Here's how the part is built. I have some questions about the finished solid (model axes, mm). A direction names the side the tool comes from. Coordinates: 2 decimals unless noted, no trailing zeros. Write each loop counter-clockwise with the first axis right and the second up, starting at its lowest first coordinate (ties: lowest second). Pieces come first, ordered by that corner, then holes. Notation, with made-up numbers: (54.5, -30) -> (68.5, -30) arc R13 ccw to (68.5, -20) -> close; hole circle Ø1 at (-1.5, -28). An arc over 180 degrees is marked (long way). Put each result on its own line as item: value. Start each with the question number.
Item 1: If we mould it in two halves opening along Y, with no side actions, what happens to faces 1 (the face through (70.768, -13.596, 0.044)), 2 (the face through (0, -9.8, 27)), 3 (the face through (1, 6, -3.175))? For each: released by +Y, released by -Y, zero draft, split by the parting line, or undercut.
Item 2: For pin 1 (9 mm diameter, centred on x = 58.5, y = -11.5, fed in from +Z) (3 decimals); pin 2 (2 mm diameter, centred on x = 60, z = 3, fed in from +Y); pin 3 (2.5 mm diameter, centred on x = 49, y = 33, fed in from +Z) (3 decimals); pin 4 (12 mm diameter, centred on x = 60.325, y = 18.775, fed in from +Z), each with a flat end and sliding along its axis, tell me the tip position at first contact or that it passes through.
Item 3: On a 3-axis mill with a long thin cutter (end or side, diameter ignored), from which of +Z, -Z, +X, -X, +Y, -Y can I reach the whole of each face in a straight line? I mean faces 4 (the face through (59, -10, 0.875)), 5 (the face through (75.59, 10.04, -1.89)), 6 (the face through (-6.133, -14.629, 25.39)). Say none if no direction works.
Item 4: I want a section at A-A, the plane z = 7. List the corners of the cut face in (x, y) for me (3 decimals).
Item 5: I want a section at B-B, the plane x = 0. List the corners of the cut face in (y, z) for me (1 decimal), then the cut area to 3 significant figures.
Item 6: I need wall thicknesses on line 1 (X direction, y = -9, z = -1); line 2 (X direction, y = -17, z = 25); line 3 (Z direction, x = 21, y = -13) (3 decimals). Which ranges of each line are inside material? Lowest first, please. Write a range as [from, to].
from build123d import *

# Parameters (mm, degrees)
BOSS_EXTRUDE1_DEPTH                              = 3.175
SKETCH2_W                                        = 31.75
SKETCH2_H                                        = 9.525
BOSS_EXTRUDE2_DEPTH                              = 47.419999902
SKETCH3_R                                        = 1.5
CUT_EXTRUDE1_DEPTH                               = 12.7
SKETCH6_R                                        = 1.5
CUT_EXTRUDE2_DEPTH                               = 12.7
SKETCH7_R                                        = 1.5
CUT_EXTRUDE3_DEPTH                               = 12.7
FILLET1_R                                        = 9.525
SKETCH12_R                                       = 7.5
CUT_EXTRUDE4_DEPTH                               = 101.032629802
CUT_EXTRUDE5_START                               = -2.54
CUT_EXTRUDE5_DEPTH                               = 2.54
FILLET3_R                                        = 1.5875
FILLET3_OF_MIRROR2_R                             = 1.5875
CBORE_FOR_M3_HEX_HEAD_MACHINE_SCREW1_D           = 3.4
CBORE_FOR_M3_HEX_HEAD_MACHINE_SCREW1_CBORE_D     = 8.4
CBORE_FOR_M3_HEX_HEAD_MACHINE_SCREW1_CBORE_DEPTH = 2.3
SKETCH19_R                                       = 4.7625
CUT_EXTRUDE6_DEPTH                               = 101.032629802


with BuildPart() as part:
    # Sketch1 → Boss-Extrude1 (new, symmetric)
    with BuildSketch(Plane.XY):
        with BuildLine():
            Line((-57.15, 44.175), (57.15, 44.175))
            ThreePointArc((57.15, 44.175), (70.620384182, 38.595384182), (76.2, 25.125))
            Line((76.2, 25.125), (76.2, -0.275))
            ThreePointArc((76.2, -0.275), (70.620384182, -13.745384182), (57.15, -19.325))
            Line((57.15, -19.325), (-57.15, -19.325))
            ThreePointArc((-57.15, -19.325), (-70.620384182, -13.745384182), (-76.2, -0.275))
            Line((-76.2, -0.275), (-76.2, 25.125))
            ThreePointArc((-76.2, 25.125), (-70.620384182, 38.595384182), (-57.15, 44.175))
        make_face()
    extrude(amount=BOSS_EXTRUDE1_DEPTH, both=True)

    # Sketch2 → Boss-Extrude2 (add)
    with BuildSketch(Plane(origin=(0, 0, 3.175), x_dir=(-1, 0, 0), z_dir=(0, 0, -1))):
        with BuildLine():
            Line((-31.75, 44.175), (31.75, 44.175))
            ThreePointArc((31.75, 44.175), (28.030256121, 35.194743879), (19.05, 31.475))
            Line((19.05, 31.475), (-19.05, 31.475))
            ThreePointArc((-19.05, 31.475), (-28.030256121, 35.194743879), (-31.75, 44.175))
        make_face()
        with Locations((0, -14.5625)):
            Rectangle(SKETCH2_W, SKETCH2_H)
    extrude(amount=-BOSS_EXTRUDE2_DEPTH)

    # Sketch3 → Cut-Extrude1 (cut)
    with BuildSketch(Plane.XY.offset(50.594999902)):
        with Locations((-20, 38.225)):
            Circle(SKETCH3_R)
        with Locations((20, 38.225)):
            Circle(SKETCH3_R)
        with Locations((-3.81, -15.515)):
            Circle(SKETCH3_R)
        with Locations((3.81, -15.515)):
            Circle(SKETCH3_R)
    extrude(amount=-CUT_EXTRUDE1_DEPTH, mode=Mode.SUBTRACT)

    # Sketch6 → Cut-Extrude2 (cut)
    with BuildSketch(Plane(origin=(0, 44.175, 0), x_dir=(1, 0, 0), z_dir=(0, 1, 0))):
        with Locations(Location((-14.85, -25.194999902, 0), (0, 0, 270))):
            Circle(SKETCH6_R)
        with Locations(Location((14.85, -25.194999902, 0), (0, 0, 90))):
            Circle(SKETCH6_R)
    extrude(amount=-CUT_EXTRUDE2_DEPTH, mode=Mode.SUBTRACT)

    # Sketch7 → Cut-Extrude3 (cut)
    with BuildSketch(Plane.XZ.offset(19.325)):
        with Locations(Location((-7.6199916, 25.194999902, 0), (0, 0, 270))):
            Circle(SKETCH7_R)
        with Locations(Location((7.6199916, 25.194999902, 0), (0, 0, 212.149655394))):
            Circle(SKETCH7_R)
    extrude(amount=-CUT_EXTRUDE3_DEPTH, mode=Mode.SUBTRACT)

    # Fillet1
    # the kernel refuses this fillet: 9.525 mm, written as the material it takes off along each edge
    with BuildSketch(Plane(origin=(-15.875, -9.8, 3.175), x_dir=(0, -1, 0), z_dir=(0, 0, 1)), Plane(origin=(15.875, -9.8, 3.175), x_dir=(-1, 0, 0), z_dir=(0, 0, 1))) as fillet1_piece_1:
        with BuildLine():
            CenterArc((FILLET1_R, FILLET1_R), FILLET1_R, 180, 90)
            Line((0, FILLET1_R), (-FILLET1_R * 0.02, FILLET1_R))
            Line((-FILLET1_R * 0.02, FILLET1_R), (-FILLET1_R * 0.02, -FILLET1_R * 0.02))
            Line((-FILLET1_R * 0.02, -FILLET1_R * 0.02), (FILLET1_R, -FILLET1_R * 0.02))
            Line((FILLET1_R, -FILLET1_R * 0.02), (FILLET1_R, 0))
        make_face()
    extrude(amount=47.419999902, mode=Mode.SUBTRACT)

    # Sketch12 → Cut-Extrude4 (cut, through all)
    with BuildSketch(Plane.XY.offset(3.175)):
        with Locations((60.325, 18.775)):
            Circle(SKETCH12_R)
        with Locations((-60.325, 18.775)):
            Circle(SKETCH12_R)
    extrude(amount=-CUT_EXTRUDE4_DEPTH, mode=Mode.SUBTRACT)

    # Sketch14 → Cut-Extrude5 (cut)
    with BuildSketch(Plane(origin=(0, 0, -3.175), x_dir=(-1, 0, 0), z_dir=(0, 0, -1)).offset(CUT_EXTRUDE5_START)):
        with BuildLine():
            ThreePointArc((-67.36426696, 21.363188685), (-66.820190528, 22.525), (-66.086070631, 23.577089669))
            Line((-66.086070631, 23.577089669), (-65.244148963, 27.295215935))
            Line((-65.244148963, 27.295215935), (-71.386034831, 29.201296117))
            ThreePointArc((-71.386034831, 29.201296117), (-75.556221789, 27.56875), (-74.88495472, 23.140989098))
            Line((-74.88495472, 23.140989098), (-70.163297927, 18.775))
            Line((-70.163297927, 18.775), (-67.36426696, 21.363188685))
        make_face()
        with BuildLine():
            Line((-65.244148963, 27.295215935), (-66.086070631, 23.577089669))
            ThreePointArc((-66.086070631, 23.577089669), (-64.075, 25.270190528), (-61.603196329, 26.165278354))
            Line((-61.603196329, 26.165278354), (-65.244148963, 27.295215935))
        make_face()
        with BuildLine():
            Line((-63.823919889, 33.567285215), (-65.244148963, 27.295215935))
            Line((-65.244148963, 27.295215935), (-61.603196329, 26.165278354))
            ThreePointArc((-61.603196329, 26.165278354), (-60.325, 26.275), (-59.046803671, 26.165278354))
            Line((-59.046803671, 26.165278354), (-55.405851037, 27.295215935))
            Line((-55.405851037, 27.295215935), (-56.826080111, 33.567285215))
            ThreePointArc((-56.826080111, 33.567285215), (-60.325, 36.3625), (-63.823919889, 33.567285215))
        make_face()
        with BuildLine():
            Line((-55.405851037, 27.295215935), (-59.046803671, 26.165278354))
            ThreePointArc((-59.046803671, 26.165278354), (-56.575, 25.270190528), (-54.563929369, 23.577089669))
            Line((-54.563929369, 23.577089669), (-55.405851037, 27.295215935))
        make_face()
        with BuildLine():
            Line((-49.263965169, 29.201296117), (-55.405851037, 27.295215935))
            Line((-55.405851037, 27.295215935), (-54.563929369, 23.577089669))
            ThreePointArc((-54.563929369, 23.577089669), (-53.829809472, 22.525), (-53.28573304, 21.363188685))
            Line((-53.28573304, 21.363188685), (-50.486702073, 18.775))
            Line((-50.486702073, 18.775), (-45.76504528, 23.140989098))
            ThreePointArc((-45.76504528, 23.140989098), (-45.093778211, 27.56875), (-49.263965169, 29.201296117))
        make_face()
        with BuildLine():
            Line((-50.486702073, 18.775), (-53.28573304, 21.363188685))
            ThreePointArc((-53.28573304, 21.363188685), (-52.941081589, 20.089438626), (-52.825, 18.775))
            ThreePointArc((-52.825, 18.775), (-52.941081589, 17.460561374), (-53.28573304, 16.186811315))
            Line((-53.28573304, 16.186811315), (-50.486702073, 18.775))
        make_face()
        with BuildLine():
            Line((-45.76504528, 14.409010902), (-50.486702073, 18.775))
            Line((-50.486702073, 18.775), (-53.28573304, 16.186811315))
            ThreePointArc((-53.28573304, 16.186811315), (-53.829809472, 15.025), (-54.563929369, 13.972910331))
            Line((-54.563929369, 13.972910331), (-55.405851037, 10.254784065))
            Line((-55.405851037, 10.254784065), (-49.263965169, 8.348703883))
            ThreePointArc((-49.263965169, 8.348703883), (-45.093778211, 9.98125), (-45.76504528, 14.409010902))
        make_face()
        with BuildLine():
            ThreePointArc((-54.563929369, 13.972910331), (-56.575, 12.279809472), (-59.046803671, 11.384721646))
            Line((-59.046803671, 11.384721646), (-55.405851037, 10.254784065))
            Line((-55.405851037, 10.254784065), (-54.563929369, 13.972910331))
        make_face()
        with BuildLine():
            Line((-61.603196329, 11.384721646), (-65.244148963, 10.254784065))
            Line((-65.244148963, 10.254784065), (-63.823919889, 3.982714785))
            ThreePointArc((-63.823919889, 3.982714785), (-60.325, 1.1875), (-56.826080111, 3.982714785))
            Line((-56.826080111, 3.982714785), (-55.405851037, 10.254784065))
            Line((-55.405851037, 10.254784065), (-59.046803671, 11.384721646))
            ThreePointArc((-59.046803671, 11.384721646), (-60.325, 11.275), (-61.603196329, 11.384721646))
        make_face()
        with BuildLine():
            ThreePointArc((-61.603196329, 11.384721646), (-64.075, 12.279809472), (-66.086070631, 13.972910331))
            Line((-66.086070631, 13.972910331), (-65.244148963, 10.254784065))
            Line((-65.244148963, 10.254784065), (-61.603196329, 11.384721646))
        make_face()
        with BuildLine():
            Line((-67.36426696, 16.186811315), (-70.163297927, 18.775))
            Line((-70.163297927, 18.775), (-74.88495472, 14.409010902))
            ThreePointArc((-74.88495472, 14.409010902), (-75.556221789, 9.98125), (-71.386034831, 8.348703883))
            Line((-71.386034831, 8.348703883), (-65.244148963, 10.254784065))
            Line((-65.244148963, 10.254784065), (-66.086070631, 13.972910331))
            ThreePointArc((-66.086070631, 13.972910331), (-66.820190528, 15.025), (-67.36426696, 16.186811315))
        make_face()
        with BuildLine():
            ThreePointArc((-67.36426696, 16.186811315), (-67.825, 18.775), (-67.36426696, 21.363188685))
            Line((-67.36426696, 21.363188685), (-70.163297927, 18.775))
            Line((-70.163297927, 18.775), (-67.36426696, 16.186811315))
        make_face()
    cut_extrude5 = extrude(amount=CUT_EXTRUDE5_DEPTH, mode=Mode.SUBTRACT)

    # Fillet3
    fillet3_edges = [part.edges().sort_by_distance(p)[0] for p in [
        (65.244148963, 27.295215935, -1.905),
        (55.405851037, 27.295215935, -1.905),
        (50.486702073, 18.775, -1.905),
        (55.405851037, 10.254784065, -1.905),
        (65.244148963, 10.254784065, -1.905),
        (70.163297927, 18.775, -1.905),
    ]]
    fillet(fillet3_edges, radius=FILLET3_R)

    # Mirror2: Cut-Extrude5 across plane
    add(cut_extrude5.mirror(Plane(origin=(0, 0, 0), x_dir=(0, 0, 1), z_dir=(1, 0, 0))), mode=Mode.SUBTRACT)

    # Fillet3 of Mirror2
    fillet3_of_mirror2_edges = [part.edges().sort_by_distance(p)[0] for p in [
        (-65.244148963, 27.295215935, -1.905),
        (-55.405851037, 27.295215935, -1.905),
        (-50.486702073, 18.775, -1.905),
        (-55.405851037, 10.254784065, -1.905),
        (-65.244148963, 10.254784065, -1.905),
        (-70.163297927, 18.775, -1.905),
    ]]
    fillet(fillet3_of_mirror2_edges, radius=FILLET3_OF_MIRROR2_R)

    # CBORE for M3 Hex Head Machine Screw1 (through all)
    with Locations(Plane.XY.offset(3.175)):
        with Locations((-47.625, 34.65), (-57.15, -9.8), (57.15, -9.8), (47.625, 34.65)):
            CounterBoreHole(CBORE_FOR_M3_HEX_HEAD_MACHINE_SCREW1_D / 2, CBORE_FOR_M3_HEX_HEAD_MACHINE_SCREW1_CBORE_D / 2, CBORE_FOR_M3_HEX_HEAD_MACHINE_SCREW1_CBORE_DEPTH)

    # Sketch19 → Cut-Extrude6 (cut, through all)
    with BuildSketch(Plane.XY.offset(3.175)):
        with Locations((0, 12.425)):
            Circle(SKETCH19_R)
    extrude(amount=-CUT_EXTRUDE6_DEPTH, mode=Mode.SUBTRACT)


solid = part.part
Calculated:
1. face 1: released by -Y
1. face 2: undercut
1. face 3: zero draft
2. pin 1: stops at z = 3.175
2. pin 2: stops at y = 44.08
2. pin 3: stops at z = 0.875
2. pin 4: passes through
3. face 4: +Z
3. face 5: -Z
3. face 6: -Y
4. outline: (-31.75, 44.175) arc R12.7 ccw to (-19.05, 31.475) -> (19.05, 31.475) arc R12.7 ccw to (31.75, 44.175) -> close; (-15.875, -19.325) -> (15.875, -19.325) arc R9.525 ccw to (6.35, -9.8) -> (-6.35, -9.8) arc R9.525 ccw to start
5. outline: (-19.3, -3.2) -> (7.7, -3.2) -> (7.7, 3.2) -> (-9.8, 3.2) -> (-9.8, 50.6) -> (-19.3, 50.6) -> close; (17.2, -3.2) -> (44.2, -3.2) -> (44.2, 50.6) -> (31.5, 50.6) -> (31.5, 3.2) -> (17.2, 3.2) -> close
5. area: 1,400 mm2
6. line 1: x = [-74.08, -58.65], [-55.65, 55.65], [58.65, 74.08]
6. line 2: x = [-15.59, -9.11], [-6.13, 6.13], [9.11, 15.59]
6. line 3: z = [-3.175, 3.175]
